The model under review builds one solid part; all positions refer to its coordinate system, in mm. Face numbers are marked on the shaded views. Coordinates: 2 decimals unless noted, no trailing zeros. Write each loop counter-clockwise with the first axis right and the second up, starting at its lowest first coordinate (ties: lowest second). Pieces come first, ordered by that corner, then holes. Notation, with made-up numbers: (63, 51) - (92, 51) arc R14 cw to (92, 77) - close; hole circle Ø3 at (32, 5.25). An arc over 180 degrees is marked (long way). Return JSON: item names as keys, results as strings. Group by question number.
(1) We need section B-B on x = -37. State the section outline as (y, z) points, then the cut area to 3 significant figures.
(2) Draft analysis for pull direction Z (two halves, no side actions). For the marked faces 1, 2, 3 and 4, state which applies: released by +Z, released by -Z, zero draft, split by the parting line, or undercut.
(3) We need section D-D on z = -37. State the section outline as (x, y) points.
(4) To check wall thickness, follow L1, parallel to X at y = 3.25, z = -35.5; L2, parallel to X at y = 7.75, z = -37; L3, parallel to Z at x = 44, y = 2. State the ranges of each line that lie inside material, in increasing order. Write a range as from..to.
(5) We need section C-C on z = 0. State the section outline as (x, y) points, then the cut area to 3 significant figures.
(6) We need section A-A on y = 4. State the section outline as (x, z) points, then the cut area to 3 significant figures.
(7) For pin 1 Ø3 at (y, z) = (3, 13.5) entering from +X; pin 2 Ø3 at (x, y) = (-39, 5.5) entering from +Z, all flat-tipped, find the tip position at first contact; note any pin that passes through.
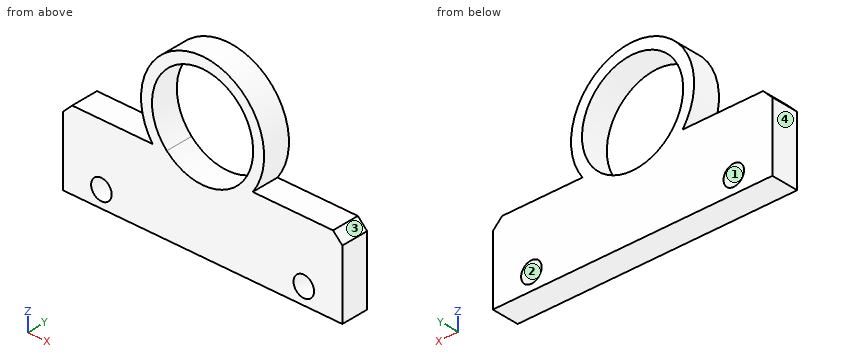
```python
from build123d import *
from build123d.topology import SkipClean

# Parameters (mm, degrees)
SKETCH1_R           = 22.5
SKETCH1_R_2         = 18.5
BOSS_EXTRUDE1_DEPTH = 10
SKETCH2_R           = 3.75
BOSS_EXTRUDE2_DEPTH = 10


with BuildPart() as part:
    # Sketch1 → Boss-Extrude1 (new body)
    with BuildSketch(Plane(origin=(0, 0, 0), x_dir=(1, 0, 0), z_dir=(0, 1, 0))):
        with Locations(Location((0, 0, 0), (0, 0, 270))):
            Circle(SKETCH1_R)
        with Locations(Location((0, 0, 0), (0, 0, 270))):
            Circle(SKETCH1_R_2, mode=Mode.SUBTRACT)
    extrude(amount=BOSS_EXTRUDE1_DEPTH)

    # Sketch2 → Boss-Extrude2 (add)
    with SkipClean():  # the faces are left unmerged after this step: merging them gives an invalid solid
        with BuildSketch(Plane(origin=(0, 0, 0), x_dir=(1, 0, 0), z_dir=(0, 1, 0))):
            with BuildLine():
                Line((18.317381325, 13.066121896), (37, 13.066121896))
                Line((37, 13.066121896), (47.681821621, 13.066121896))
                Line((47.681821621, 13.066121896), (51.096419029, 16.480719304))
                Line((51.096419029, 16.480719304), (51.096419029, 41.480719304))
                Line((51.096419029, 41.480719304), (0, 41.480719304))
                Line((0, 41.480719304), (-51.096419029, 41.480719304))
                Line((-51.096419029, 41.480719304), (-51.096419029, 16.480719304))
                Line((-51.096419029, 16.480719304), (-47.681821621, 13.066121896))
                Line((-47.681821621, 13.066121896), (-37, 13.066121896))
                Line((-37, 13.066121896), (-18.317381325, 13.066121896))
                Line((-18.317381325, 13.066121896), (-13.096811009, 13.066121896))
                ThreePointArc((-13.096811009, 13.066121896), (0, 18.5), (13.096811009, 13.066121896))
                Line((13.096811009, 13.066121896), (18.317381325, 13.066121896))
            make_face()
            with Locations(Location((-37, 35.387659732, 0), (0, 0, 270))):
                Circle(SKETCH2_R, mode=Mode.SUBTRACT)
            with Locations(Location((37, 35.387659732, 0), (0, 0, 270))):
                Circle(SKETCH2_R, mode=Mode.SUBTRACT)
        extrude(amount=BOSS_EXTRUDE2_DEPTH)


solid = part.part
```
Ans:
{
 "1": {"outline": "(0, -41.48) - (10, -41.48) - (10, -39.14) - (0, -39.14) - close; (0, -31.64) - (10, -31.64) - (10, -13.07) - (0, -13.07) - close", "area": "209 mm²"},
 "2": {"face 1": "undercut", "face 2": "undercut", "face 3": "released by +Z", "face 4": "zero draft"},
 "3": {"outline": "(-51.1, 0) - (-40.39, 0) - (-40.39, 10) - (-51.1, 10) - close; (-33.61, 0) - (33.61, 0) - (33.61, 10) - (-33.61, 10) - close; (40.39, 0) - (51.1, 0) - (51.1, 10) - (40.39, 10) - close"},
 "4": {"L1": "-51.1..-40.75, -33.25..33.25, 40.75..51.1", "L2": "-51.1..-40.39, -33.61..33.61, 40.39..51.1", "L3": "-41.48..-13.07"},
 "5": {"outline": "(-22.5, 0) - (-18.5, 0) - (-18.5, 10) - (-22.5, 10) - close; (18.5, 0) - (22.5, 0) - (22.5, 10) - (18.5, 10) - close", "area": "80.0 mm²"},
 "6": {"outline": "(-51.1, -41.48) - (51.1, -41.48) - (51.1, -16.48) - (47.68, -13.07) - (18.32, -13.07) arc R22.5 ccw (long way) to (-18.32, -13.07) - (-47.68, -13.07) - (-51.1, -16.48) - close; hole circle Ø7.5 at (-37, -35.39); hole circle Ø37 at (0, 0); hole circle Ø7.5 at (37, -35.39)", "area": "3,080 mm²"},
 "7": {"pin 1": "x = 19.03", "pin 2": "z = -13.07"}
}
